from build123d import *

# Parameters (mm, degrees)
SKETCH1_W           = 116
SKETCH1_H           = 93
SKETCH1_R           = 4.25
BOSS_EXTRUDE1_DEPTH = 5


with BuildPart() as part:
    # Sketch1 → Boss-Extrude1 (new body)
    with BuildSketch(Plane.XY):
        Rectangle(SKETCH1_W, SKETCH1_H)
        with Locations((-43, 36.5)):
            Circle(SKETCH1_R, mode=Mode.SUBTRACT)
        with Locations((43, 36.5)):
            Circle(SKETCH1_R, mode=Mode.SUBTRACT)
        with Locations((43, -36.5)):
            Circle(SKETCH1_R, mode=Mode.SUBTRACT)
        with Locations((-43, -36.5)):
            Circle(SKETCH1_R, mode=Mode.SUBTRACT)
        with Locations((0, 36.5)):
            Circle(SKETCH1_R, mode=Mode.SUBTRACT)
    extrude(amount=BOSS_EXTRUDE1_DEPTH)


solid = part.part
Geometry check sheet. Reference: the model listing, model coordinates, mm. Give positions to 0.01 mm unless a question says otherwise; leave off trailing zeros. Order: outer loops, then holes, each group sorted by start corner. A loop starts at its lowest first (then second) coordinate and runs counter-clockwise, first axis right, second up.
1. Depth check by flat-ended pin: pin 1 (13.5 mm diameter, centred on x = 0, y = 36.5, fed in from +Z). Enter the tip coordinate at first touch or a pass-through.
Completed:
pin 1: stops at z = 5
2. Draft check along Y on faces 1 (the face through (-1, 1, 5)), 2 (the face through (-1, 46.5, 2)), 3 (the face through (-47.246, -36.313, 2.465)). Enter one of: pulls with the +Y half, pulls with the -Y half, needs draft (parallel to the pull), parting line crosses it, or undercut.
Completed:
face 1: needs draft
face 2: pulls with the +Y half
face 3: undercut
3. Scan lines: line 1 (Y direction, x = 43, z = 3.4); line 2 (Y direction, x = -44, z = 3.2); line 3 (Y direction, x = -3.5, z = 1.4). Record each from-to range of solid material in increasing order.
Completed:
line 1: y = -46.5 to -40.75, -32.25 to 32.25, 40.75 to 46.5
line 2: y = -46.5 to -40.63, -32.37 to 32.37, 40.63 to 46.5
line 3: y = -46.5 to 34.09, 38.91 to 46.5
4. Sectioned sample at A-A (x = -43). Record the boundary of the cut face in (y, z).
Completed:
outline: (-46.5, 0) - (-40.75, 0) - (-40.75, 5) - (-46.5, 5) - close; (-32.25, 0) - (32.25, 0) - (32.25, 5) - (-32.25, 5) - close; (40.75, 0) - (46.5, 0) - (46.5, 5) - (40.75, 5) - close
5. Sectioned sample at D-D (y = 36.5). Record the boundary of the cut face in (x, z), then the cut area to 4 significant figures.
Completed:
outline: (-58, 0) - (-47.25, 0) - (-47.25, 5) - (-58, 5) - close; (-38.75, 0) - (-4.25, 0) - (-4.25, 5) - (-38.75, 5) - close; (4.25, 0) - (38.75, 0) - (38.75, 5) - (4.25, 5) - close; (47.25, 0) - (58, 0) - (58, 5) - (47.25, 5) - close
area: 452.5 mm2
6. Sectioned sample at B-B (y = -36.5). Record the boundary of the cut face in (x, z).
Completed:
outline: (-58, 0) - (-47.25, 0) - (-47.25, 5) - (-58, 5) - close; (-38.75, 0) - (38.75, 0) - (38.75, 5) - (-38.75, 5) - close; (47.25, 0) - (58, 0) - (58, 5) - (47.25, 5) - close
7. Sectioned sample at C-C (x = 0). Record the boundary of the cut face in (y, z).
Completed:
outline: (-46.5, 0) - (32.25, 0) - (32.25, 5) - (-46.5, 5) - close; (40.75, 0) - (46.5, 0) - (46.5, 5) - (40.75, 5) - close
